Input: dimensioned drawing with shaded views. Units: mm. Origin: part minimum x, y, z. Coordinates: 2 decimals unless noted, no trailing zeros. Order: outer loops, then holes, each group sorted by start corner. A loop starts at its lowest first (then second) coordinate and runs counter-clockwise, first axis right, second up. Notation, with made-up numbers: (-22.75, -35.5) -> (-15.75, -35.5) arc R15 ccw to (-15.75, -18.5) -> close; hole circle Ø1 at (37.5, -2). An arc over 180 degrees is marked (long way). Answer as CSV lines item,"result".
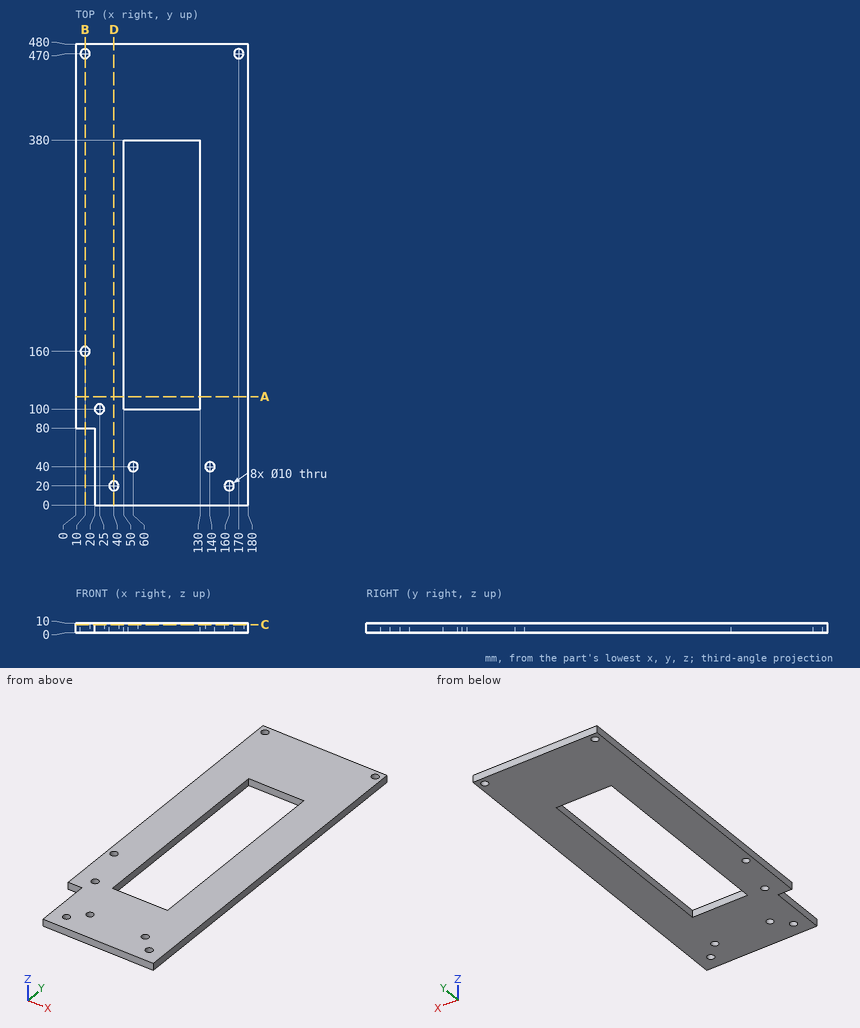
1. Cut plane B-B (x = 10). Return the cut outline in (y, z), plus the area to 3 significant figures.
Findings:
outline,"(80, 0) -> (155, 0) -> (155, 10) -> (80, 10) -> close; (165, 0) -> (465, 0) -> (465, 10) -> (165, 10) -> close; (475, 0) -> (480, 0) -> (480, 10) -> (475, 10) -> close"
area,"3,800 mm2"
2. Contact query for a flat-ended pin moving along its axis: pin 1 (5 mm diameter, centred on x = 12, z = 6.5, fed in from -Y). Output: stop coordinate, or through.
Findings:
pin 1,"stops at y = 80"
3. Cut plane C-C (z = 8.5). State how many separate pieces and enclosed holes the cut face has, plus the area to 3 significant figures.
Findings:
separate pieces,"1"
enclosed holes,"9"
area,"61,800 mm2"
4. Ray query, line 1 along X through (y, z) = (470, 4.5); line 2 along Y through (x, z) = (40, 4.75); line 3 along Y through (x, z) = (10, 5). Return the intervals inside material, ascending.
Findings:
line 1,"x = 0 to 5, 15 to 165, 175 to 180"
line 2,"y = 0 to 15, 25 to 480"
line 3,"y = 80 to 155, 165 to 465, 475 to 480"
5. Cut plane D-D (x = 40). Return the cut outline in (y, z).
Findings:
outline,"(0, 0) -> (15, 0) -> (15, 10) -> (0, 10) -> close; (25, 0) -> (480, 0) -> (480, 10) -> (25, 10) -> close"
6. Cut plane A-A (y = 113). Return the cut outline in (x, z), plus the area to 3 significant figures.
Findings:
outline,"(0, 0) -> (50, 0) -> (50, 10) -> (0, 10) -> close; (130, 0) -> (180, 0) -> (180, 10) -> (130, 10) -> close"
area,"1,000 mm2"
